Input: part model. Units: mm. Frame: model coordinates. A direction names the side the tool comes from. Give positions to 0.01 mm unless a question says otherwise; leave off trailing zeros. Loops run counter-clockwise (first coordinate to the right, second up) from the corner with the lowest first, then second, coordinate; pieces in that order, holes last. Notation, with made-up numbers: (61, -6) - (80, -6) arc R9 ccw to (80, 5) - close; hole circle Ø10 at (44.5, 8.25). An arc over 180 degrees is marked (long way). One line per item, written item: value.
from build123d import *

# Parameters (mm, degrees)
F0_R          = 20
F0_R_2        = 15.237
F1_DEPTH      = 77
F3_R          = 6.065714741
F4_DEPTH      = 25
F4_DEPTH_BACK = 25
F3_W          = 11.689950712
F3_H          = 6.0669332743
F5_DEPTH      = 25
F5_DEPTH_BACK = 25


# Not quite as in the source:
# - a fillet or chamfer that OpenCascade refuses, or shapes differently, is made with other operations: its cross-section is extruded or revolved along the edge and cut away or added


with BuildPart() as f1:
    # F0 (on Top) → F1 (new body)
    with BuildSketch(Plane.XY):
        Circle(F0_R)
        with Locations((0, 1.5118854353)):
            Circle(F0_R_2, mode=Mode.SUBTRACT)
    extrude(amount=F1_DEPTH)

    # F2: fillet of radius 5 on 1 edges, made by hand

    # F2_s1 → F2_t2 (revolve, cut)
    with BuildSketch(Plane.XZ):
        with BuildLine():
            ThreePointArc((20, 72), (18.5355339059, 75.5355339059), (15, 77))
            Line((15, 77), (20, 77))
            Line((20, 77), (20, 72))
        make_face()
    revolve(axis=Axis((0, 0, 77), (0, 0, 1)), mode=Mode.SUBTRACT)

    # F3 (on Right) → F4 (join, two sides)
    with BuildSketch(Plane.YZ) as f4_sk:
        with Locations((0, 34.2814810574)):
            Circle(F3_R)
    extrude(amount=F4_DEPTH)
    extrude(f4_sk.sketch, amount=-F4_DEPTH_BACK)

    # F3 (on Right) → F5 (cut, two sides)
    with BuildSketch(Plane.YZ) as f5_sk:
        with Locations((0, 34.2814810574)):
            Circle(F3_R)
        with Locations((0.5918950774, 61.7306679487)):
            Rectangle(F3_W, F3_H)
    extrude(amount=-F5_DEPTH, mode=Mode.SUBTRACT)
    extrude(f5_sk.sketch, amount=F5_DEPTH_BACK, mode=Mode.SUBTRACT)


solid = f1.part
Item 1: Material intervals for L1, parallel to Y at x = 0, z = 57.5; L2, parallel to Z at x = -18, y = 0; L3, parallel to X at y = -9.5, z = 25, sorted ascending.
Verdict:
L1: y = -20 to -13.73, 16.75 to 20
L2: z = 0 to 28.22, 40.35 to 58.7, 64.76 to 76
L3: x = -17.6 to -10.53, 10.53 to 17.6
Item 2: Section A-A, the plane y = 0. Output: boundary loops of the cut face in (x, z).
Verdict:
outline: (-20, 0) - (-15.16, 0) - (-15.16, 28.22) - (-20, 28.22) - close; (-20, 40.35) - (-15.16, 40.35) - (-15.16, 58.7) - (-20, 58.7) - close; (-20, 64.76) - (-15.16, 64.76) - (-15.16, 77) arc R5 ccw to (-20, 72) - close; (15.16, 0) - (20, 0) - (20, 28.22) - (15.16, 28.22) - close; (15.16, 40.35) - (20, 40.35) - (20, 58.7) - (15.16, 58.7) - close; (15.16, 64.76) - (20, 64.76) - (20, 72) arc R5 ccw to (15.16, 77) - close
Item 3: Section C-C, the plane z = 38. Output: boundary loops of the cut face in (x, y), and give its area (3 significant figures).
Verdict:
outline: (-19.42, -4.79) arc R20 ccw to (19.42, -4.79) - (13.87, -4.79) arc R15.24 cw to (-13.87, -4.79) - close; (-19.42, 4.79) - (-14.88, 4.79) arc R15.24 cw to (14.88, 4.79) - (19.42, 4.79) arc R20 ccw to start
area: 433 mm^2
Item 4: Draft query along Z for faces 3 (the face through (-16, -5.253, 62)), 4 (the face through (-17, 6.437, 62)), 5 (the face through (0, -14, 77)), 6 (the face through (-6, -13, 0)). Return one class per face: pulls with the +Z half, pulls with the -Z half, needs draft (parallel to the pull), parting line crosses it, or undercut.
Verdict:
face 3: undercut
face 4: undercut
face 5: pulls with the +Z half
face 6: pulls with the -Z half
Item 5: Section B-B, the plane x = 0. Output: boundary loops of the cut face in (y, z), and give its area (3 significant figures).
Verdict:
outline: (-20, 0) - (-13.73, 0) - (-13.73, 77) - (-15, 77) arc R5 ccw to (-20, 72) - close; (16.75, 0) - (20, 0) - (20, 72) arc R5 ccw to (16.75, 76.68) - close
area: 723 mm^2
Item 6: Pin query (flat end, axial travel): P1, Ø1.9, axis at x = 18, y = -1, coming from the +Z side; P2, Ø5, axis at x = -16.5, z = 62, coming from the -Y side; P3, Ø3, axis at x = -16, z = 63, coming from the +Y side (3 decimals). Return the tip coordinate at first contact, or that it passes through.
Verdict:
P1: stops at z = 76.55
P2: stops at y = -14.28
P3: stops at y = 13.775
Item 7: Section D-D, the plane z = 24.5. Output: boundary loops of the cut face in (x, y), and give its area (3 significant figures).
Verdict:
outline: circle Ø40 at (0, 0); hole circle Ø30.47 at (0, 1.51)
area: 527 mm^2
Item 8: Access query for faces 1 (the face through (17, 1, 64.764)), 2 (the face through (18.475, -7.66, 35.496)). Directions: +Z, -Z, +X, -X, +Y, -Y. A direction counts if a zero-diameter tool reaches every point of the face in a straight line with its end or side. Return the directions, or none.
Verdict:
face 1: +X, -X
face 2: +Z, -Z
